Check sheet for the modelled part. Datum: model origin and axes. Units: mm. Face numbers are marked on the shaded views. Round coordinates to 2 decimals unless told otherwise and drop trailing zeros. Write each loop counter-clockwise with the first axis right and the second up, starting at its lowest first coordinate (ties: lowest second). Pieces come first, ordered by that corner, then holes. Notation, with made-up numbers: M 78.5,32 L 83.5,32 A15 ccw 83.5,56 Z; hole C -27,55 d7. An arc over 180 degrees is marked long. Answer in a Markdown table with one row per item.
```python
from build123d import *

# Parameters (mm, degrees)
PAD_DEPTH    = 10
SKETCH001_R  = 1.5
PAD001_DEPTH = 10


with BuildPart() as part:
    # Sketch → Pad (new body)
    with BuildSketch(Plane.XY):
        Polygon((74.568908, 0), (0, 0), (46.488009, 99.693857), (55.551087, 95.467674), (15.696856, 10), (74.568908, 10), align=None)
    extrude(amount=PAD_DEPTH)

    # Sketch001 (on Face4 of Pad) → Pad001 (join)
    with BuildSketch(Plane(origin=(9.063078, -4.226183, 0), x_dir=(0.422618, 0.906308, 0), z_dir=(0.906308, -0.422618, 0))):
        with BuildLine():
            Line((110, 10), (100, 10))
            Line((100, 10), (100, 20))
            ThreePointArc((110, 20), (105, 25), (100, 20))
            Line((110, 10), (110, 20))
        make_face()
        with Locations((105, 20)):
            Circle(SKETCH001_R, mode=Mode.SUBTRACT)
        with BuildLine():
            Line((45, 10), (45, 20))
            ThreePointArc((45, 20), (40, 25), (35, 20))
            Line((35, 10), (35, 20))
            Line((45, 10), (35, 10))
        make_face()
        with Locations((40, 20)):
            Circle(SKETCH001_R, mode=Mode.SUBTRACT)
    extrude(amount=-PAD001_DEPTH)


solid = part.part
```
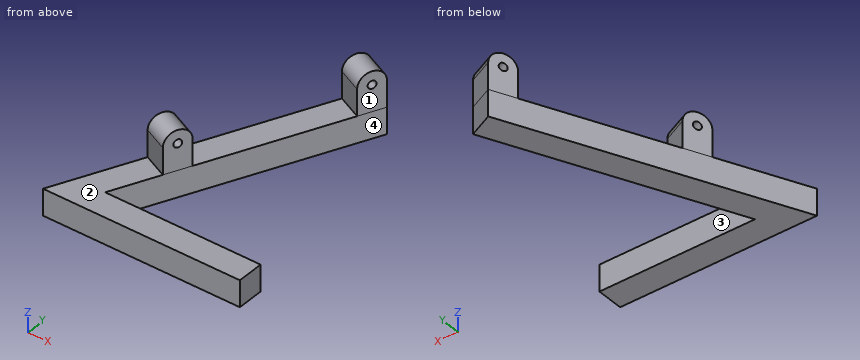
1. Section check B-B, the plane x = 41. Record the cut outline in (y, z).
Found:
| item | result |
|---|---|
| outline | M 0,0 L 10,0 L 10,10 L 0,10 Z; M 64.26,0 L 87.92,0 L 87.92,10 L 64.26,10 Z |
2. Draft check along Y on the marked faces 1, 2, 3 and 4. Enter one of: +Y half, -Y half, draft (parallel to the pull), parting line (faces both ways), or undercut.
Found:
| item | result |
|---|---|
| face 1 | -Y half |
| face 2 | draft |
| face 3 | undercut |
| face 4 | undercut |
3. Section check A-A, the plane z = 14.25. Record the cut outline in (x, y), and give its area (3 significant figures).
Found:
| item | result |
|---|---|
| outline | M 14.79,31.72 L 23.85,27.49 L 28.08,36.56 L 19.02,40.78 Z; M 42.26,90.63 L 51.32,86.4 L 55.55,95.47 L 46.49,99.69 Z |
| area | 200 mm2 |
4. Section check C-C, the plane z = 7.5. Record the cut outline in (x, y).
Found:
| item | result |
|---|---|
| outline | M 0,0 L 74.57,0 L 74.57,10 L 15.7,10 L 55.55,95.47 L 46.49,99.69 Z |
5. Go/stop test with flat-tipped pins: pin 1 (11 mm diameter, centred on x = 44, z = 5, fed in from +Y); pin 2 (4 mm diameter, centred on x = 48, z = 20.5, fed in from -Y); pin 3 (2 mm diameter, centred on x = 54.5, z = 22, fed in from -Y). Record where each tip stops, or that it passes through.
Found:
| item | result |
|---|---|
| pin 1 | stops at y = 99.69 |
| pin 2 | stops at y = 87.04 |
| pin 3 | stops at y = 91.07 |
6. Scan lines: L1, parallel to Z at x = 19, y = 26.5; L2, parallel to Y at x = 19.5, z = 6.75; L3, parallel to Y at x = 21.5, z = 7.75. Record each from-to range of solid material in increasing order.
Found:
| item | result |
|---|---|
| L1 | z = 0 to 10 |
| L2 | y = 0 to 10, 18.16 to 41.82 |
| L3 | y = 0 to 10, 22.44 to 46.11 |
7. Section check D-D, the plane x = 67.5. Record the cut outline in (y, z), and give its area (3 significant figures).
Found:
| item | result |
|---|---|
| outline | M 0,0 L 10,0 L 10,10 L 0,10 Z |
| area | 100 mm2 |
